Autodesk Inventor part; units mm, degrees
ref_plane "YZ Plane" through (0, 0, 0) normal (1, 0, 0) x (0, 1, 0)
ref_plane "XZ Plane" through (0, 0, 0) normal (0, 1, 0) x (-1, 0, 0)
ref_plane "XY Plane" through (0, 0, 0) normal (0, 0, 1) x (1, 0, 0)
sketch "Sketch1" plane through (0, 0, 0) normal (0, 0, 1) x (1, 0, 0)
  circle A0 centre (0, 0) radius 20
  circle A1 centre (0, 0) radius 35
  dimension "d0" = 70
  dimension "d1" = 40
extrude "Extrusion1" add sketch "Sketch1" along normal blind 3
sketch "Sketch2" plane through (0, 0, 3) normal (0, 0, 1) x (1, 0, 0)
  circle A0 centre (0, 0) radius 23.75 construction
  circle A1 centre (0, 0) radius 32 construction
  point P0 (23.75, 0)
  point P1 (32, 0)
  dimension "d4" = 64
  dimension "d5" = 47.5
hole "Hole1" at (23.75, 0, 3) at (32, 0, 3) direction (0, 0, -1) diameter 3.2 end through all
pattern_circular "Circular Pattern1" count 4 over 360 about axis through (0, 0, 0) along (0, 0, 1) of "Hole1"
properties part number "plasma_chamber_holder" material "Copper"
Geometry check sheet. Reference: the model listing, model coordinates, mm. Coordinates: 2 decimals unless noted, no trailing zeros. Loops run counter-clockwise (first coordinate to the right, second up) from the corner with the lowest first, then second, coordinate; pieces in that order, holes last.
Item 1: Sectioned sample at D-D, the plane y = -23.75. Record the boundary of the cut face in (x, z), then the cut area to 3 significant figures.
Item 2: Sectioned sample at B-B, the plane x = -11. Record the boundary of the cut face in (y, z), then the cut area to 3 significant figures.
Item 3: Release check for a two-part mould opening along Y. For faces 1 (the face through (-22.164, -0.208, 1.479)), 2 (the face through (-28, 21, 1)), 3 (the face through (15, -15, 3)) record: released by +Y, released by -Y, zero draft, split by the parting line, or undercut.
Item 4: Go/stop test with flat-tipped pins: pin 1 Ø2.5 at (x, y) = (0, 32) entering from +Z; pin 2 Ø1.5 at (y, z) = (-23.5, 0.5) entering from +X; pin 3 Ø1 at (y, z) = (27, 1) entering from +X. Record where each tip stops, or that it passes through.
Item 5: Sectioned sample at A-A, the plane y = 0. Record the boundary of the cut face in (x, z), then the cut area to 3 significant figures.
Item 6: Sectioned sample at C-C, the plane z = 2.35. Count the separate pieces of the cut face and the enclosed holes in it, then the cut area to 3 significant figures.
Item 7: Thickness scan on line 1 (Y direction, x = 0, z = 1.5); line 2 (Y direction, x = 1, z = 1.5); line 3 (Y direction, x = 23, z = 0.3). Record the ranges inside material, lowest first.
Check result:
1. outline: (-25.71, 0) - (-1.6, 0) - (-1.6, 3) - (-25.71, 3) - close; (1.6, 0) - (25.71, 0) - (25.71, 3) - (1.6, 3) - close
1. area: 145 mm2
2. outline: (-33.23, 0) - (-16.7, 0) - (-16.7, 3) - (-33.23, 3) - close; (16.7, 0) - (33.23, 0) - (33.23, 3) - (16.7, 3) - close
2. area: 99.1 mm2
3. face 1: undercut
3. face 2: split by the parting line
3. face 3: zero draft
4. pin 1: passes through
4. pin 2: stops at x = 26.6
4. pin 3: stops at x = 22.86
5. outline: (-35, 0) - (-33.6, 0) - (-33.6, 3) - (-35, 3) - close; (-30.4, 0) - (-25.35, 0) - (-25.35, 3) - (-30.4, 3) - close; (-22.15, 0) - (-20, 0) - (-20, 3) - (-22.15, 3) - close; (20, 0) - (22.15, 0) - (22.15, 3) - (20, 3) - close; (25.35, 0) - (30.4, 0) - (30.4, 3) - (25.35, 3) - close; (33.6, 0) - (35, 0) - (35, 3) - (33.6, 3) - close
5. area: 51.6 mm2
6. separate pieces: 1
6. enclosed holes: 9
6. area: 2,530 mm2
7. line 1: y = -35 to -33.6, -30.4 to -25.35, -22.15 to -20, 20 to 22.15, 25.35 to 30.4, 33.6 to 35
7. line 2: y = -34.99 to -33.25, -30.75 to -25, -22.5 to -19.97, 19.97 to 22.5, 25 to 30.75, 33.25 to 34.99
7. line 3: y = -26.38 to -1.41, 1.41 to 26.38
